Part model, mm, in its own coordinate system. A direction names the side the tool comes from. Round coordinates to 2 decimals unless told otherwise and drop trailing zeros. Order: outer loops, then holes, each group sorted by start corner. A loop starts at its lowest first (then second) coordinate and runs counter-clockwise, first axis right, second up. Notation, with made-up numbers: M 46,32.25 L 53,32.25 A17 cw 53,59.25 Z; hole C 56,72.25 d9. An arc over 180 degrees is marked long. Write each question's results on one line, items separated by ' | '. Start each with the question number.
1. Two-plate mould, pull along X, no slides. Class faces 3 (the face through (31, 0, 10)), 4 (the face through (75, 0, 5)), 5 (the face through (-6, 0, 5)): +X half, -X half, draft (parallel to the pull), parting line (faces both ways), or undercut.
2. Band-saw the part on D-D, the plane y = 12. List the corners of the cut face in (x, z).
3. Drop flat-ended pins along their axis: pin 1 Ø3 at (x, y) = (33, -7) entering from +Z; pin 2 Ø5 at (x, z) = (19, 13) entering from +Y; pin 3 Ø8 at (y, z) = (-8, 13) entering from -X. Give the stop position or say it passes through.
4. Band-saw the part on B-B, the plane y = 3. List the corners of the cut face in (x, z).
5. Probe L1, parallel to Y at x = 0, z = 4.5; L2, parallel to Z at x = 37, y = -11; L3, parallel to X at y = 2, z = 6.75. List the from-to ranges inside material, lowest first. Write a range as [from, to].
6. Band-saw the part on A-A, the plane z = 5.25. List the corners of the cut face in (x, y), then the cut area to 3 significant figures.
7. Which spindle directions (+Z, -Z, +X, -X, +Y, -Y) get a long thin tool onto all of the face, cutting with end or side? Do faces 1 (the face through (30, -15, 5)), 2 (the face through (54, 0, 15)). Say none if no direction does.
8. Band-saw the part on C-C, the plane x = 29. List the corners of the cut face in (y, z).
```python
from build123d import *

# Parameters (mm, degrees)
CROQUIS1_R              = 6
SALIENTE_EXTRUIR1_DEPTH = 10
CROQUIS2_R              = 6
SALIENTE_EXTRUIR2_DEPTH = 10


with BuildPart() as part:
    # Croquis1 → Saliente-Extruir1 (new body)
    with BuildSketch(Plane.XY):
        with BuildLine():
            Line((0, 15), (60, 15))
            ThreePointArc((60, 15), (75, 0), (60, -15))
            Line((60, -15), (0, -15))
            ThreePointArc((0, -15), (-15, 0), (0, 15))
        make_face()
        Circle(CROQUIS1_R, mode=Mode.SUBTRACT)
    extrude(amount=SALIENTE_EXTRUIR1_DEPTH)

    # Croquis2 → Saliente-Extruir2 (add)
    with BuildSketch(Plane.XY.offset(10)):
        with Locations((60, 0)):
            Circle(CROQUIS2_R)
    extrude(amount=SALIENTE_EXTRUIR2_DEPTH)


solid = part.part
```
Solution:
1) face 3: draft | face 4: +X half | face 5: undercut
2) outline: M -9,0 L 69,0 L 69,10 L -9,10 Z
3) pin 1: z = 10 | pin 2: through | pin 3: x = -14.01
4) outline: M -14.7,0 L -5.2,0 L -5.2,10 L -14.7,10 Z; M 5.2,0 L 74.7,0 L 74.7,10 L 65.2,10 L 65.2,20 L 54.8,20 L 54.8,10 L 5.2,10 Z
5) L1: [-15, -6], [6, 15] | L2: [0, 10] | L3: [-14.87, -5.66], [5.66, 74.87]
6) outline: M 0,-15 L 60,-15 A15 ccw 60,15 L 0,15 A15 ccw Z; hole C 0,0 d12 | area: 2,390 mm^2
7) face 1: +Z, -Z, +X, -X, -Y | face 2: +Z
8) outline: M -15,0 L 15,0 L 15,10 L -15,10 Z
